from build123d import *
from build123d.topology import SkipClean

# Parameters (mm, degrees)
SKETCH1_R            = 38
SKETCH1_R_2          = 35
SKETCH1_R_3          = 2
BOSS_EXTRUDE6_DEPTH  = 2
SKETCH1_7_R          = 38
SKETCH1_7_R_2        = 35
BOSS_EXTRUDE7_DEPTH  = 24
BOSS_EXTRUDE8_DEPTH  = 24
CIRPATTERN1_COUNT    = 28
BOSS_EXTRUDE9_DEPTH  = 24
SKETCH4_R            = 1.85
CUT_EXTRUDE2_DEPTH   = 4
BOSS_EXTRUDE12_DEPTH = 9
SKETCH7_R            = 1.5
CUT_EXTRUDE4_DEPTH   = 9
BOSS_EXTRUDE17_DEPTH = 24
SKETCH11_10_R        = 1.9
CUT_EXTRUDE7_DEPTH   = 24
CIRPATTERN2_COUNT    = 4
SKETCH5_W            = 41.086585788
SKETCH5_H            = 115.80999181
CUT_EXTRUDE3_DEPTH   = 24


with BuildPart() as part:
    # Sketch1 → Boss-Extrude6 (new body)
    # profile 1 of 5: a face of its own
    with BuildSketch(Plane(origin=(0, 0, 0), x_dir=(1, 0, 0), z_dir=(0, 1, 0))):
        with Locations(Location((0, 0, 0), (0, 0, 270))):
            Circle(SKETCH1_R)
        Circle(SKETCH1_R_2, mode=Mode.SUBTRACT)
    # profile 2 of 5: a face of its own
    with BuildSketch(Plane(origin=(0, 0, 0), x_dir=(1, 0, 0), z_dir=(0, 1, 0))):
        with BuildLine():
            Line((1, 33), (0, 33))
            Line((0, 33), (-1, 33))
            Line((-1, 33), (-2.5, 34.910600109))
            ThreePointArc((-2.5, 34.910600109), (-23.848480035, -25.617376915), (35, 0))
            ThreePointArc((35, 0), (25.617376915, 23.848480035), (2.5, 34.910600109))
            Line((2.5, 34.910600109), (1, 33))
        make_face()
        Circle(SKETCH1_R_3, mode=Mode.SUBTRACT)
    # profile 3 of 5: a face of its own
    with BuildSketch(Plane(origin=(0, 0, 0), x_dir=(1, 0, 0), z_dir=(0, 1, 0))):
        Circle(SKETCH1_R_3)
    # profile 4 of 5: a face of its own
    with BuildSketch(Plane(origin=(0, 0, 0), x_dir=(1, 0, 0), z_dir=(0, 1, 0))):
        with BuildLine():
            Line((0, 33), (0, 35))
            ThreePointArc((0, 35), (-1.250798979, 34.977642887), (-2.5, 34.910600109))
            Line((-2.5, 34.910600109), (-1, 33))
            Line((-1, 33), (0, 33))
        make_face()
    # profile 5 of 5: a face of its own
    with BuildSketch(Plane(origin=(0, 0, 0), x_dir=(1, 0, 0), z_dir=(0, 1, 0))):
        with BuildLine():
            ThreePointArc((2.5, 34.910600109), (1.250798979, 34.977642887), (0, 35))
            Line((0, 35), (0, 33))
            Line((0, 33), (1, 33))
            Line((1, 33), (2.5, 34.910600109))
        make_face()
    extrude(amount=BOSS_EXTRUDE6_DEPTH)

    # Sketch1<7> → Boss-Extrude7 (add)
    with BuildSketch(Plane(origin=(0, 0, 0), x_dir=(1, 0, 0), z_dir=(0, 1, 0))):
        with Locations(Location((0, 0, 0), (0, 0, 270))):
            Circle(SKETCH1_7_R)
        with Locations(Location((0, 0, 0), (0, 0, 270))):
            Circle(SKETCH1_7_R_2, mode=Mode.SUBTRACT)
    extrude(amount=BOSS_EXTRUDE7_DEPTH)

    # Sketch1<8> → Boss-Extrude8 (add)
    with BuildSketch(Plane(origin=(0, 0, 0), x_dir=(1, 0, 0), z_dir=(0, 1, 0))):
        with BuildLine():
            ThreePointArc((2.5, 34.910600109), (1.250798979, 34.977642887), (0, 35))
            Line((0, 35), (0, 33))
            Line((0, 33), (1, 33))
            Line((1, 33), (2.5, 34.910600109))
        make_face()
        with BuildLine():
            Line((0, 33), (0, 35))
            ThreePointArc((0, 35), (-1.250798979, 34.977642887), (-2.5, 34.910600109))
            Line((-2.5, 34.910600109), (-1, 33))
            Line((-1, 33), (0, 33))
        make_face()
    boss_extrude8 = extrude(amount=BOSS_EXTRUDE8_DEPTH)

    # CirPattern1: Boss-Extrude8 ×28 about axis
    cirpattern1_axis = Axis((0, 0, 0), (0, 1, 0))
    for i in range(1, CIRPATTERN1_COUNT):
        add(boss_extrude8.rotate(cirpattern1_axis, i * 360 / CIRPATTERN1_COUNT))

    # Sketch3 → Boss-Extrude9 (add)
    with BuildSketch(Plane(origin=(0, 0, 0), x_dir=(1, 0, 0), z_dir=(0, 1, 0))):
        with BuildLine():
            Line((0, -38), (0, -53))
            Line((0, -53), (4, -53))
            Line((4, -53), (4, -40.780878967))
            Line((4, -40.780878967), (7.535533906, -37.245345062))
            ThreePointArc((7.535533906, -37.245345062), (3.786613768, -37.810865583), (0, -38))
        make_face()
    boss_extrude9 = extrude(amount=BOSS_EXTRUDE9_DEPTH)

    # Sketch4 → Cut-Extrude2 (cut)
    with BuildSketch(Plane(origin=(0, 0, 0), x_dir=(0, 0, -1), z_dir=(1, 0, 0))):
        with Locations(Location((-46.890439484, 5, 0), (0, 0, 180))):
            Circle(SKETCH4_R)
        with Locations(Location((-46.890439484, 19, 0), (0, 0, 180))):
            Circle(SKETCH4_R)
    cut_extrude2 = extrude(amount=CUT_EXTRUDE2_DEPTH, mode=Mode.SUBTRACT)

    # Mirror1: Boss-Extrude9, Cut-Extrude2 across plane
    add(boss_extrude9.mirror(Plane.XY))
    add(cut_extrude2.mirror(Plane.XY), mode=Mode.SUBTRACT)

    # Sketch6 → Boss-Extrude12 (add)
    with BuildSketch(Plane(origin=(0, 0, 0), x_dir=(1, 0, 0), z_dir=(0, 1, 0))):
        Polygon((0, 6.870468203), (-5.95, 3.435234102), (-5.95, -3.435234102), (0, -6.870468203), (5.95, -3.435234102), (5.95, 3.435234102), align=None)
    extrude(amount=BOSS_EXTRUDE12_DEPTH)

    # Sketch7 → Cut-Extrude4 (cut)
    with BuildSketch(Plane(origin=(0, 0, 0), x_dir=(1, 0, 0), z_dir=(0, 1, 0))):
        with Locations(Location((0, 0, 0), (0, 0, 270))):
            Circle(SKETCH7_R)
    extrude(amount=CUT_EXTRUDE4_DEPTH, mode=Mode.SUBTRACT)

    # Sketch11 → Boss-Extrude17 (add)
    with BuildSketch(Plane(origin=(0, 0, 0), x_dir=(1, 0, 0), z_dir=(0, 1, 0))):
        with BuildLine():
            ThreePointArc((25.493387139, 28.179553087), (27.575155537, 28.634381073), (28.770057685, 26.870057685))
            ThreePointArc((28.770057685, 26.870057685), (28.61620219, 26.121072126), (28.179553087, 25.493387139))
            ThreePointArc((28.179553087, 25.493387139), (29.185469438, 24.335331798), (30.143828836, 23.137622676))
            ThreePointArc((30.143828836, 23.137622676), (29.69848481, 29.69848481), (23.137622676, 30.143828836))
            ThreePointArc((23.137622676, 30.143828836), (24.335331798, 29.185469438), (25.493387139, 28.179553087))
        make_face()
    boss_extrude17 = extrude(amount=BOSS_EXTRUDE17_DEPTH)

    # Sketch11<10> → Cut-Extrude7 (cut)
    with SkipClean():  # the faces are left unmerged after this step: merging them gives an invalid solid
        with BuildSketch(Plane(origin=(0, 0, 0), x_dir=(1, 0, 0), z_dir=(0, 1, 0))):
            with Locations(Location((26.870057685, 26.870057685, 0), (0, 0, 270))):
                Circle(SKETCH11_10_R)
        cut_extrude7 = extrude(amount=CUT_EXTRUDE7_DEPTH, mode=Mode.SUBTRACT)

    # CirPattern2: Boss-Extrude17, Cut-Extrude7 ×4 about axis
    with SkipClean():  # the faces are left unmerged after this step: merging them gives an invalid solid
        cirpattern2_axis = Axis((0, 0, 0), (0, 1, 0))
        add([boss_extrude17.rotate(cirpattern2_axis, i * 360 / CIRPATTERN2_COUNT) for i in range(1, CIRPATTERN2_COUNT)])
        add([cut_extrude7.rotate(cirpattern2_axis, i * 360 / CIRPATTERN2_COUNT) for i in range(1, CIRPATTERN2_COUNT)], mode=Mode.SUBTRACT)

    # Sketch5 → Cut-Extrude3 (cut)
    with SkipClean():  # the faces are left unmerged after this step: merging them gives an invalid solid
        with BuildSketch(Plane(origin=(0, 0, 0), x_dir=(1, 0, 0), z_dir=(0, 1, 0))):
            with Locations((-20.543292894, -1.918879007)):
                Rectangle(SKETCH5_W, SKETCH5_H)
        extrude(amount=CUT_EXTRUDE3_DEPTH, mode=Mode.SUBTRACT)


solid = part.part
Work out the finished part from the listing and answer in its coordinate system (mm). A direction names the side the tool comes from. Round coordinates to 2 decimals unless told otherwise and drop trailing zeros. Write each loop counter-clockwise with the first axis right and the second up, starting at its lowest first coordinate (ties: lowest second). Pieces come first, ordered by that corner, then holes. Notation, with made-up numbers: M 72,-21.5 L 123,-21.5 A24 ccw 123,-6.5 Z; hole C 68.25,23.25 d11. An arc over 180 degrees is marked long. Use a Markdown table: item, result.
1) Determine the mould class of faces 4 (the face through (1.76, 12.85, 33.97)), 5 (the face through (1.972, 17.44, 47.885)), 6 (the face through (9.28, 12.85, 32.73)), 7 (the face through (14.306, 12.846, -29.738)) for opening direction X: pulls with the +X half, pulls with the -X half, needs draft (parallel to the pull), parting line crosses it, or undercut.
Taken from the geometry:
| item | result |
|---|---|
| face 4 | undercut |
| face 5 | needs draft |
| face 6 | undercut |
| face 7 | pulls with the -X half |
2) The part is cut by section B-B on y = 19. State how many separate pieces and enclosed holes the cut face has, plus the area to 3 significant figures.
Taken from the geometry:
| item | result |
|---|---|
| separate pieces | 3 |
| enclosed holes | 2 |
| area | 581 mm2 |
3) The part is cut by section D-D on z = 46. Give the vertices of the cut face in (x, y).
Taken from the geometry:
| item | result |
|---|---|
| outline | M 0,0 L 4,0 L 4,3.38 L 0,3.38 Z; M 0,6.62 L 4,6.62 L 4,17.38 L 0,17.38 Z; M 0,20.62 L 4,20.62 L 4,24 L 0,24 Z |
4) Consider line 1 (Z direction, x = 26, y = 13.75); line 2 (Z direction, x = 34.5, y = 6); line 3 (Z direction, x = 30, y = 10.75). Determine where each line is inside the solid, lowest interval first. Write a range as [from, to].
Taken from the geometry:
| item | result |
|---|---|
| line 1 | z = [-31.16, -28.56], [-25.18, -20.32], [20.32, 25.18], [28.56, 31.16] |
| line 2 | z = [-15.93, -5.37], [-2.18, 2.18], [5.37, 15.93] |
| line 3 | z = [-29.37, -18.03], [-16.65, -13.76], [13.76, 16.65], [18.03, 29.37] |
5) Flat-ended cylindrical pins translate along their axes: pin 1 (1.8 mm diameter, centred on x = 3, z = 1, fed in from +Y); pin 2 (4.5 mm diameter, centred on y = 19, z = 46.89, fed in from +X); pin 3 (5 mm diameter, centred on x = 22.5, y = 17, fed in from -Z). Find the tip coordinate at first contact, or state that the pin passes through.
Taken from the geometry:
| item | result |
|---|---|
| pin 1 | stops at y = 9 |
| pin 2 | stops at x = 4 |
| pin 3 | stops at z = -32.31 |
6) Which of the six approach directions +Z, -Z, +X, -X, +Y, -Y give full straight-line access (tool end or side, diameter ignored) to faces 1 (the face through (0, 9, 39)), 2 (the face through (25.45, 12.85, 22.52)), 3 (the face through (11.58, 12.85, -33.03))?
Taken from the geometry:
| item | result |
|---|---|
| face 1 | +Z, -Z, -X, +Y, -Y |
| face 2 | -X, +Y |
| face 3 | +Y |
7) The part is cut by section A-A on z = 0. Give the vertices of the cut face in (x, y).
Taken from the geometry:
| item | result |
|---|---|
| outline | M 1.5,0 L 38,0 L 38,24 L 33,24 L 33,2 L 5.95,2 L 5.95,9 L 1.5,9 Z |
